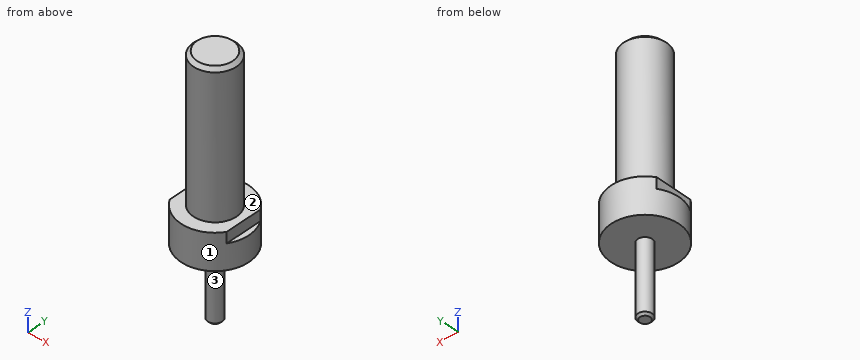
```python
from build123d import *

# Parameters (mm, degrees)
SKETCH_1_R          = 1
EXTRUDE_1_DEPTH     = 10
SKETCH_2_R          = 4.75
EXTRUDE_2_DEPTH     = 5
CUT_EXTRUDE_1_DEPTH = 1.5
SKETCH_4_W          = 2.580322654
SKETCH_4_H          = 8.195778588
CUT_EXTRUDE_3_DEPTH = 1.5
SKETCH_5_R          = 3
EXTRUDE_3_DEPTH     = 20
CHAMFER_1_SIZE      = 0.5
CHAMFER_2_SIZE      = 0.3


with BuildPart() as part:
    # Эскиз1 → Вытянуть1 (new body)
    with BuildSketch(Plane.XY):
        Circle(SKETCH_1_R)
    extrude(amount=EXTRUDE_1_DEPTH)

    # Эскиз2 → Вытянуть2 (add)
    with BuildSketch(Plane.XY.offset(10)):
        with Locations(Location((0, 0, 0), (0, 0, 212.636897504))):
            Circle(SKETCH_2_R)
    extrude(amount=EXTRUDE_2_DEPTH)

    # Эскиз3 → Вырез-Вытянуть1 (cut)
    with BuildSketch(Plane.XY.offset(15)):
        with BuildLine():
            Line((-4, 3.641620684), (-4, -3.641620684))
            ThreePointArc((-4, -3.641620684), (-5.409380852, 0), (-4, 3.641620684))
        make_face()
    extrude(amount=-CUT_EXTRUDE_1_DEPTH, mode=Mode.SUBTRACT)

    # Эскиз4 → Вырез-Вытянуть3 (cut)
    with BuildSketch(Plane.XY.offset(15)):
        with Locations((5.290161327, 0.120888876)):
            Rectangle(SKETCH_4_W, SKETCH_4_H)
    extrude(amount=-CUT_EXTRUDE_3_DEPTH, mode=Mode.SUBTRACT)

    # Эскиз5 → Вытянуть3 (add)
    with BuildSketch(Plane.XY.offset(15)):
        Circle(SKETCH_5_R)
    extrude(amount=EXTRUDE_3_DEPTH)

    # Фаска1
    chamfer_1_edges = [part.edges().sort_by_distance(p)[0] for p in [
        (-3, 0, 35),
    ]]
    chamfer(chamfer_1_edges, length=CHAMFER_1_SIZE)

    # Фаска2
    chamfer_2_edges = [part.edges().sort_by_distance(p)[0] for p in [
        (-1, 0, 0),
    ]]
    chamfer(chamfer_2_edges, length=CHAMFER_2_SIZE)


solid = part.part
```
Verification items for the finished model (mm, model axes). Face numbers are marked on the shaded views. A direction names the side the tool comes from. Give positions to 0.01 mm unless a question says otherwise; leave off trailing zeros. Order: outer loops, then holes, each group sorted by start corner. A loop starts at its lowest first (then second) coordinate and runs counter-clockwise, first axis right, second up. Notation, with made-up numbers: M -14,4 L 20,4 A25 ccw 20,18 Z; hole C 23.5,55 d11. An arc over 180 degrees is marked long. Answer in a Markdown table with one row per item. Add a question column.
Item 1: Section check D-D, the plane y = 4. Enter the section's corners in (x, z).
Item 2: Scan lines: probe 1 along Z at (x, y) = (1.5, 2); probe 2 along Z at (x, y) = (1.5, 3.25); probe 3 along X at (y, z) = (-4, 13). Record each from-to range of solid material in increasing order. Write a range as from..to.
Item 3: Section check B-B, the plane x = 0. Enter the section's corners in (y, z).
Item 4: Gauge pin test, flat ends, axial feed: pin 1 (2 mm diameter, centred on y = 1.5, z = 17.5, fed in from +X); pin 2 (1.5 mm diameter, centred on y = -2, z = 5, fed in from +X); pin 3 (2 mm diameter, centred on y = -3, z = 27, fed in from -X); pin 4 (1 mm diameter, centred on x = -3.5, z = 11, fed in from +Y). Record the tip position at first contact, or that the pin passes through.
Item 5: Section check A-A, the plane y = 0. Enter the section's corners in (x, z).
Item 6: Section check C-C, the plane z = 13. Enter the section's corners in (x, y).
Item 7: Tool access check on the marked faces 1, 2 and 3. Record the directions out of +Z, -Z, +X, -X, +Y, -Y that give a thin tool (end or side, any length) a straight path to the whole face; none if there is none.
Filled sheet:
| question | item | result |
|---|---|---|
| 1 | outline | M -2.56,10 L 2.56,10 L 2.56,15 L -2.56,15 Z |
| 2 | probe 1 | z = 10..35 |
| 2 | probe 2 | z = 10..15 |
| 2 | probe 3 | x = -2.56..2.56 |
| 3 | outline | M -4.75,10 L -1,10 L -1,0.3 L -0.7,0 L 0.7,0 L 1,0.3 L 1,10 L 4.75,10 L 4.75,15 L 3,15 L 3,34.5 L 2.5,35 L -2.5,35 L -3,34.5 L -3,15 L -4.75,15 Z |
| 4 | pin 1 | stops at x = 2.96 |
| 4 | pin 2 | passes through |
| 4 | pin 3 | stops at x = -2.24 |
| 4 | pin 4 | stops at y = 3.68 |
| 5 | outline | M -4.75,10 L -1,10 L -1,0.3 L -0.7,0 L 0.7,0 L 1,0.3 L 1,10 L 4.75,10 L 4.75,13.5 L 4,13.5 L 4,15 L 3,15 L 3,34.5 L 2.5,35 L -2.5,35 L -3,34.5 L -3,15 L -4,15 L -4,13.5 L -4.75,13.5 Z |
| 6 | outline | C 0,0 d9.5 |
| 7 | face 1 | +Z, -Z |
| 7 | face 2 | +Z |
| 7 | face 3 | -Z |
